The listing builds one solid part. Answer for the finished solid, in the listing's coordinates (mm). Round coordinates to 2 decimals unless told otherwise and drop trailing zeros. Order: outer loops, then holes, each group sorted by start corner. A loop starts at its lowest first (then second) coordinate and runs counter-clockwise, first axis right, second up. Notation, with made-up numbers: (43.25, -27) - (76.25, -27) arc R12 ccw to (76.25, -17) - close; hole circle Ø7 at (-30, 33). An arc over 180 degrees is marked (long way). Write item = value, one per line.
from build123d import *

# Parameters (mm, degrees)
FILLET1_R           = 2.54
SKETCH3_R           = 33.455795103
SKETCH3_R_2         = 19.05
CUT_EXTRUDE1_DEPTH  = 5.08
SKETCH4_R           = 12.7
BOSS_EXTRUDE1_DEPTH = 5.08
SKETCH5_R           = 7.62
CUT_EXTRUDE2_DEPTH  = 2.54
FILLET6_R           = 1.27
REVOLVE2_ANGLE      = 180
SCALE1_SCALE        = 0.5


with BuildPart() as part:
    # Sketch1 → Revolve1 (revolve)
    with BuildSketch(Plane.XY, mode=Mode.PRIVATE) as revolve1_sk:
        Polygon((0, 0), (0, -25.4), (60.96, -25.4), (35.56, 0), align=None)
    revolve(revolve1_sk.sketch.rotate(Axis((0, 0, 0), (0, -1, 0)), 180), axis=Axis((0, 0, 0), (0, -1, 0)))

    # Fillet1
    fillet1_edges = [part.edges().sort_by_distance(p)[0] for p in [
        (35.56, 0, 0),
    ]]
    fillet(fillet1_edges, radius=FILLET1_R)

    # Sketch3 → Cut-Extrude1 (cut)
    with BuildSketch(Plane(origin=(0, 0, 0), x_dir=(1, 0, 0), z_dir=(0, 1, 0))):
        with Locations(Location((0, 0, 0), (0, 0, 180))):
            Circle(SKETCH3_R)
        with Locations(Location((0, 0, 0), (0, 0, 180))):
            Circle(SKETCH3_R_2, mode=Mode.SUBTRACT)
    extrude(amount=-CUT_EXTRUDE1_DEPTH, mode=Mode.SUBTRACT)

    # Fillet4: read off the stored shape, not the designer's step
    # Fillet4 outline → Fillet4 (revolve, cut)
    with BuildSketch(Plane.XY):
        with BuildLine():
            ThreePointArc((33.455795103, -2.058582249), (33.73406349, -0.902654003), (34.507897552, 0))
            Line((34.507897552, 0), (33.455795103, 0))
            Line((33.455795103, 0), (33.455795103, -2.058582249))
        make_face()
    revolve(axis=Axis((0, 0, 0), (0, 1, 0)), mode=Mode.SUBTRACT)

    # Sketch4 → Boss-Extrude1 (add)
    with BuildSketch(Plane(origin=(0, 0, 0), x_dir=(1, 0, 0), z_dir=(0, 1, 0))):
        Circle(SKETCH4_R)
    extrude(amount=BOSS_EXTRUDE1_DEPTH)

    # Sketch5 → Cut-Extrude2 (cut)
    with BuildSketch(Plane(origin=(0, 5.08, 0), x_dir=(1, 0, 0), z_dir=(0, 1, 0))):
        with Locations(Location((0, 0, 0), (0, 0, 180))):
            Circle(SKETCH5_R)
    extrude(amount=-CUT_EXTRUDE2_DEPTH, mode=Mode.SUBTRACT)

    # Fillet6
    fillet6_edges = [part.edges().sort_by_distance(p)[0] for p in [
        (19.05, -5.08, 0),
    ]]
    fillet(fillet6_edges, radius=FILLET6_R)

    # Sketch6 → Revolve2 (revolve)
    with BuildSketch(Plane(origin=(0, 2.54, 0), x_dir=(1, 0, 0), z_dir=(0, 1, 0))):
        with BuildLine():
            Line((0, -3.81), (0, 3.81))
            ThreePointArc((0, 3.81), (-3.81, 0), (0, -3.81))
        make_face()
    revolve(axis=Axis((0, 2.54, 3.81), (0, 0, -1)), revolution_arc=REVOLVE2_ANGLE)


with BuildPart() as part_1:
    # Scale1: scaled about (0, -15.502710002, 0)
    add(part.part.scale(SCALE1_SCALE).moved(Location((0, -7.751355001, 0))))


solid = part_1.part
Q1. Find the intervals of material crossed by line 1 (Z direction, x = 0.5, y = -6.25); line 2 (X direction, y = -8.5, z = 3); line 3 (Z direction, x = 0, y = -9.15) (3 decimals), in increasing order. Write a range as from..to.
Model answer:
line_1 = -6.33..-3.78, -1.82..1.82, 3.78..6.33
line_2 = -18.28..-16.49, -9.04..9.04, 16.49..18.28
line_3 = -19.179..-16.728, -9.525..9.525, 16.728..19.179
Q2. Determine the mould class of faces 1 (the face through (-1.38, -6.5, 6.2)), 2 (the face through (0, -20.451, 0)), 3 (the face through (0.496, -5.837, 3.778)) for opening direction X: released by +X, released by -X, zero draft, split by the parting line, or undercut.
Model answer:
face_1 = split by the parting line
face_2 = zero draft
face_3 = undercut
Q3. Section A-A on z = 0 is taken. Determine the outline of the cut face in (x, y) (3 decimals).
Model answer:
outline = (-30.48, -20.451) - (30.48, -20.451) - (18.152, -8.123) arc R1.27 ccw to (17.254, -7.751) arc R1.27 ccw to (16.728, -8.781) - (16.728, -10.291) - (10.16, -10.291) arc R0.635 cw to (9.525, -9.656) - (9.525, -7.751) - (6.35, -7.751) - (6.35, -5.211) - (3.81, -5.211) - (3.81, -6.481) - (1.905, -6.481) arc R1.905 ccw to (-1.905, -6.481) - (-3.81, -6.481) - (-3.81, -5.211) - (-6.35, -5.211) - (-6.35, -7.751) - (-9.525, -7.751) - (-9.525, -9.656) arc R0.635 cw to (-10.16, -10.291) - (-16.728, -10.291) - (-16.728, -8.781) arc R1.27 ccw to (-17.254, -7.751) arc R1.27 ccw to (-18.152, -8.123) - close
Q4. Section C-C on y = -17.75 is taken. Determine the outline of the cut face in (x, z), then the cut area to 3 significant figures.
Model answer:
outline = circle Ø55.56 at (0, 0)
area = 2,420 mm^2
Q5. Section D-D on y = -13 is taken. Determine the outline of the cut face in (x, z).
Model answer:
outline = circle Ø46.06 at (0, 0)
Q6. Flat-ended cylindrical pins translate along their axes: P1, Ø5.5, axis at x = -3.5, z = -4, coming from the +Y side; P2, Ø5, axis at x = -22.5, y = -18.5, coming from the +Z side; P3, Ø4, axis at x = -2.5, z = -1.5, coming from the +Y side. Find the tip coordinate at first contact, or state that the pin passes through.
Model answer:
P1 = -5.21
P2 = 22.15
P3 = -4.81
Q7. Section B-B on x = 0 is taken. Determine the outline of the cut face in (y, z) (3 decimals), then the cut area to 3 significant figures.
Model answer:
outline = (-20.451, -30.48) - (-8.123, -18.152) arc R1.27 ccw to (-7.751, -17.254) arc R1.27 ccw to (-8.781, -16.728) - (-10.291, -16.728) - (-10.291, -10.16) arc R0.635 cw to (-9.656, -9.525) - (-7.751, -9.525) - (-7.751, -6.35) - (-5.211, -6.35) - (-5.211, -3.81) - (-6.481, -3.81) - (-6.481, -1.905) arc R1.905 ccw to (-6.481, 1.905) - (-6.481, 3.81) - (-5.211, 3.81) - (-5.211, 6.35) - (-7.751, 6.35) - (-7.751, 9.525) - (-9.656, 9.525) arc R0.635 cw to (-10.291, 10.16) - (-10.291, 16.728) - (-8.781, 16.728) arc R1.27 ccw to (-7.751, 17.254) arc R1.27 ccw to (-8.123, 18.152) - (-20.451, 30.48) - close
area = 604 mm^2
